For this review, take the finished solid that the model builds, in its own axes (mm). A direction names the side the tool comes from. Coordinates: 2 decimals unless noted, no trailing zeros. Write each loop counter-clockwise with the first axis right and the second up, starting at its lowest first coordinate (ties: lowest second). Pieces come first, ordered by that corner, then holes.
1) We need section C-C on z = 19. Give the number of separate pieces and of enclosed holes in the cut face, then the cut area to 3 significant figures.
2) We need section A-A on x = 13.5. Write out the cut boundary in (y, z).
3) Mouldability with a two-part tool opening along X and no side actions: class faces 4 (the face through (-28, 30.241, 12)), 5 (the face through (-17, 0, 69)), 6 (the face through (10.102, -12.325, 89.716)) as pulls with the +X half, pulls with the -X half, needs draft (parallel to the pull), parting line crosses it, or undercut.
4) Insertion check: P1, Ø8, axis at y = -30.5, z = 80.5, coming from the +X side; P2, Ø5.5, axis at y = 27.5, z = 18.5, coming from the +X side; P3, Ø3, axis at y = 24, z = 7, coming from the +X side; P4, Ø0.9, axis at x = -30.5, z = 13.5, coming from the +Y side. Each pin has a flat end and moves straight along its axis. Give the tip position at first contact, or say it passes through.
5) For faces 1 (the face through (-16.186, 25, 12)), 2 (the face through (8.91, -12.32, 36.75)), 3 (the face through (45.226, -17.865, 21.044)), list the 3-axis set-ups (+Z, -Z, +X, -X, +Y, -Y) from which the entire face can be reached by the end or side of a thin tool; tool diameter is ignored.
6) We need section D-D on x = -56.5. Write out the cut boundary in (y, z).
7) To check wall thickness, follow line 1 along Y through (x, z) = (-20.5, 15.5); line 2 along Y through (x, z) = (-66, 95); line 3 along Z through (x, y) = (0.5, 16). State the ranges of each line that lie inside material, in increasing order.
8) We need section B-B on y = -23. Write out the cut boundary in (x, z), then the cut area to 3 significant figures.
from build123d import *

# Parameters (mm, degrees)
F0_W     = 1.1385447797
F0_H     = 10.6680987737
F1_DEPTH = 25
F3_DEPTH = 25


with BuildPart() as f1:
    # F0 (on Top) → F1 (new body)
    with BuildSketch(Plane.XY):
        Polygon((0, -46.6304384172), (46.141307801, -17.2826088965), (-5.3850366841, -15.2486749252), align=None)
        Polygon((-32.335957761, 9.7168054916), (-37.6630462706, 40.7608710229), (-71.6585168016, 12.759203091), align=None)
        Polygon((46.141307801, -17.2826088965), (37.9891358316, 38.1521731615), (-9.3640666491, 7.9394637296), (-5.3850366841, -15.2486749252), align=None)
        Polygon((-5.3850366841, -15.2486749252), (-28.2065235078, -14.347827062), (-61.4673942327, -46.6304384172), (0, -46.6304384172), align=None)
        Polygon((-28.2065235078, -14.347827062), (-32.335957761, 9.7168054916), (-71.6585168016, 12.759203091), (-61.4673942327, -46.6304384172), align=None)
        Polygon((37.9891358316, 38.1521731615), (-37.6630462706, 40.7608710229), (-32.335957761, 9.7168054916), (-9.3640666491, 7.9394637296), align=None)
        Polygon((-29.9031199126, 24.5017413181), (-29.9031199126, 20.217390731), (-31.0679894271, 20.217390731), (-31.0679894271, 30.2405335024), (-25.4805644678, 30.2405335024), (-25.4805644678, 29.2050939339), (-29.9031199126, 29.2050939339), (-29.9031199126, 25.5371808865), (-25.7481992715, 25.5371808865), (-25.7481992715, 24.5017413181), align=None, mode=Mode.SUBTRACT)
        with BuildLine():
            Line((-18.5286407553, 20.217390731), (-19.3732259965, 20.217390731))
            Line((-19.3732259965, 20.217390731), (-19.5991799701, 21.2879299458))
            Line((-19.5991799701, 21.2879299458), (-19.6540231676, 21.2879299458))
            add(Edge.make_bspline(
                [(-19.6540231676, 21.2879299458), (-20.2156175098, 20.5815495622), (-20.7739212601, 20.3303677178)],
                knots=[0, 0, 0, 1, 1, 1], degree=2))
            add(Edge.make_bspline(
                [(-20.7739212601, 20.3303677178), (-21.3322250105, 20.0791858733), (-22.1702290679, 20.0791858733)],
                knots=[0, 0, 0, 1, 1, 1], degree=2))
            add(Edge.make_bspline(
                [(-22.1702290679, 20.0791858733), (-23.2868365686, 20.0791858733), (-23.9208239315, 20.6561363108)],
                knots=[0, 0, 0, 1, 1, 1], degree=2))
            add(Edge.make_bspline(
                [(-23.9208239315, 20.6561363108), (-24.5548112944, 21.2330867483), (-24.5548112944, 22.2948510515)],
                knots=[0, 0, 0, 1, 1, 1], degree=2))
            add(Edge.make_bspline(
                [(-24.5548112944, 22.2948510515), (-24.5548112944, 24.569746883), (-20.9154167096, 24.6794332779)],
                knots=[0, 0, 0, 1, 1, 1], degree=2))
            Line((-20.9154167096, 24.6794332779), (-19.6408608002, 24.721114108))
            Line((-19.6408608002, 24.721114108), (-19.6408608002, 25.1883781505))
            add(Edge.make_bspline(
                [(-19.6408608002, 25.1883781505), (-19.6408608002, 26.0724504939), (-20.0203757267, 26.4936462506)],
                knots=[0, 0, 0, 1, 1, 1], degree=2))
            add(Edge.make_bspline(
                [(-20.0203757267, 26.4936462506), (-20.3998906533, 26.9148420072), (-21.2378947108, 26.9148420072)],
                knots=[0, 0, 0, 1, 1, 1], degree=2))
            add(Edge.make_bspline(
                [(-21.2378947108, 26.9148420072), (-22.1768102516, 26.9148420072), (-23.3614233172, 26.3400852976)],
                knots=[0, 0, 0, 1, 1, 1], degree=2))
            Line((-23.3614233172, 26.3400852976), (-23.7124197811, 27.2109952736))
            add(Edge.make_bspline(
                [(-23.7124197811, 27.2109952736), (-23.1574066226, 27.5115359958), (-22.495997661, 27.6826467719)],
                knots=[0, 0, 0, 1, 1, 1], degree=2))
            add(Edge.make_bspline(
                [(-22.495997661, 27.6826467719), (-21.8345886994, 27.853757548), (-21.167695418, 27.853757548)],
                knots=[0, 0, 0, 1, 1, 1], degree=2))
            add(Edge.make_bspline(
                [(-21.167695418, 27.853757548), (-19.8251339437, 27.853757548), (-19.1768873495, 27.2581604234)],
                knots=[0, 0, 0, 1, 1, 1], degree=2))
            add(Edge.make_bspline(
                [(-19.1768873495, 27.2581604234), (-18.5286407553, 26.6625632988), (-18.5286407553, 25.3463265593)],
                knots=[0, 0, 0, 1, 1, 1], degree=2))
            Line((-18.5286407553, 25.3463265593), (-18.5286407553, 20.217390731))
        make_face(mode=Mode.SUBTRACT)
        with BuildLine():
            add(Edge.make_bspline(
                [(-15.0471945793, 26.7305688637), (-14.2530650798, 27.853757548), (-12.6889370877, 27.853757548)],
                knots=[0, 0, 0, 1, 1, 1], degree=2))
            add(Edge.make_bspline(
                [(-12.6889370877, 27.853757548), (-11.2081707557, 27.853757548), (-10.3888133854, 26.8424489865)],
                knots=[0, 0, 0, 1, 1, 1], degree=2))
            add(Edge.make_bspline(
                [(-10.3888133854, 26.8424489865), (-9.569456015, 25.831140425), (-9.569456015, 23.981827806)],
                knots=[0, 0, 0, 1, 1, 1], degree=2))
            add(Edge.make_bspline(
                [(-9.569456015, 23.981827806), (-9.569456015, 22.1303214591), (-10.3953945691, 21.1047536662)],
                knots=[0, 0, 0, 1, 1, 1], degree=2))
            add(Edge.make_bspline(
                [(-10.3953945691, 21.1047536662), (-11.2213331231, 20.0791858733), (-12.6889370877, 20.0791858733)],
                knots=[0, 0, 0, 1, 1, 1], degree=2))
            add(Edge.make_bspline(
                [(-12.6889370877, 20.0791858733), (-13.4238359339, 20.0791858733), (-14.030401698, 20.3501112689)],
                knots=[0, 0, 0, 1, 1, 1], degree=2))
            add(Edge.make_bspline(
                [(-14.030401698, 20.3501112689), (-14.6369674621, 20.6210366644), (-15.0471945793, 21.1848247345)],
                knots=[0, 0, 0, 1, 1, 1], degree=2))
            Line((-15.0471945793, 21.1848247345), (-15.1305562395, 21.1848247345))
            Line((-15.1305562395, 21.1848247345), (-15.3696725805, 20.217390731))
            Line((-15.3696725805, 20.217390731), (-16.185739359, 20.217390731))
            Line((-16.185739359, 20.217390731), (-16.185739359, 30.8854895047))
            Line((-16.185739359, 30.8854895047), (-15.0471945793, 30.8854895047))
            Line((-15.0471945793, 30.8854895047), (-15.0471945793, 28.2925031279))
            add(Edge.make_bspline(
                [(-15.0471945793, 28.2925031279), (-15.0471945793, 27.4215931519), (-15.1020377768, 26.7305688637)],
                knots=[0, 0, 0, 1, 1, 1], degree=2))
            Line((-15.1020377768, 26.7305688637), (-15.0471945793, 26.7305688637))
        make_face(mode=Mode.SUBTRACT)
        with BuildLine():
            Line((1.4342831273, 20.217390731), (0.5896978861, 20.217390731))
            Line((0.5896978861, 20.217390731), (0.3637439125, 21.2879299458))
            Line((0.3637439125, 21.2879299458), (0.308900715, 21.2879299458))
            add(Edge.make_bspline(
                [(0.308900715, 21.2879299458), (-0.2526936272, 20.5815495622), (-0.8109973775, 20.3303677178)],
                knots=[0, 0, 0, 1, 1, 1], degree=2))
            add(Edge.make_bspline(
                [(-0.8109973775, 20.3303677178), (-1.3693011279, 20.0791858733), (-2.2073051853, 20.0791858733)],
                knots=[0, 0, 0, 1, 1, 1], degree=2))
            add(Edge.make_bspline(
                [(-2.2073051853, 20.0791858733), (-3.323912686, 20.0791858733), (-3.9579000489, 20.6561363108)],
                knots=[0, 0, 0, 1, 1, 1], degree=2))
            add(Edge.make_bspline(
                [(-3.9579000489, 20.6561363108), (-4.5918874118, 21.2330867483), (-4.5918874118, 22.2948510515)],
                knots=[0, 0, 0, 1, 1, 1], degree=2))
            add(Edge.make_bspline(
                [(-4.5918874118, 22.2948510515), (-4.5918874118, 24.569746883), (-0.952492827, 24.6794332779)],
                knots=[0, 0, 0, 1, 1, 1], degree=2))
            Line((-0.952492827, 24.6794332779), (0.3220630824, 24.721114108))
            Line((0.3220630824, 24.721114108), (0.3220630824, 25.1883781505))
            add(Edge.make_bspline(
                [(0.3220630824, 25.1883781505), (0.3220630824, 26.0724504939), (-0.0574518441, 26.4936462506)],
                knots=[0, 0, 0, 1, 1, 1], degree=2))
            add(Edge.make_bspline(
                [(-0.0574518441, 26.4936462506), (-0.4369667707, 26.9148420072), (-1.2749708282, 26.9148420072)],
                knots=[0, 0, 0, 1, 1, 1], degree=2))
            add(Edge.make_bspline(
                [(-1.2749708282, 26.9148420072), (-2.213886369, 26.9148420072), (-3.3984994346, 26.3400852976)],
                knots=[0, 0, 0, 1, 1, 1], degree=2))
            Line((-3.3984994346, 26.3400852976), (-3.7494958985, 27.2109952736))
            add(Edge.make_bspline(
                [(-3.7494958985, 27.2109952736), (-3.19448274, 27.5115359958), (-2.5330737784, 27.6826467719)],
                knots=[0, 0, 0, 1, 1, 1], degree=2))
            add(Edge.make_bspline(
                [(-2.5330737784, 27.6826467719), (-1.8716648168, 27.853757548), (-1.2047715354, 27.853757548)],
                knots=[0, 0, 0, 1, 1, 1], degree=2))
            add(Edge.make_bspline(
                [(-1.2047715354, 27.853757548), (0.1377899389, 27.853757548), (0.7860365331, 27.2581604234)],
                knots=[0, 0, 0, 1, 1, 1], degree=2))
            add(Edge.make_bspline(
                [(0.7860365331, 27.2581604234), (1.4342831273, 26.6625632988), (1.4342831273, 25.3463265593)],
                knots=[0, 0, 0, 1, 1, 1], degree=2))
            Line((1.4342831273, 25.3463265593), (1.4342831273, 20.217390731))
        make_face(mode=Mode.SUBTRACT)
        with Locations((-7.0126661485, 25.5514401179)):
            Rectangle(F0_W, F0_H, mode=Mode.SUBTRACT)
        with BuildLine():
            add(Edge.make_bspline(
                [(4.9157293033, 26.7305688637), (5.7098588028, 27.853757548), (7.2739867949, 27.853757548)],
                knots=[0, 0, 0, 1, 1, 1], degree=2))
            add(Edge.make_bspline(
                [(7.2739867949, 27.853757548), (8.7547531269, 27.853757548), (9.5741104972, 26.8424489865)],
                knots=[0, 0, 0, 1, 1, 1], degree=2))
            add(Edge.make_bspline(
                [(9.5741104972, 26.8424489865), (10.3934678676, 25.831140425), (10.3934678676, 23.981827806)],
                knots=[0, 0, 0, 1, 1, 1], degree=2))
            add(Edge.make_bspline(
                [(10.3934678676, 23.981827806), (10.3934678676, 22.1303214591), (9.5675293135, 21.1047536662)],
                knots=[0, 0, 0, 1, 1, 1], degree=2))
            add(Edge.make_bspline(
                [(9.5675293135, 21.1047536662), (8.7415907595, 20.0791858733), (7.2739867949, 20.0791858733)],
                knots=[0, 0, 0, 1, 1, 1], degree=2))
            add(Edge.make_bspline(
                [(7.2739867949, 20.0791858733), (6.5390879487, 20.0791858733), (5.9325221846, 20.3501112689)],
                knots=[0, 0, 0, 1, 1, 1], degree=2))
            add(Edge.make_bspline(
                [(5.9325221846, 20.3501112689), (5.3259564205, 20.6210366644), (4.9157293033, 21.1848247345)],
                knots=[0, 0, 0, 1, 1, 1], degree=2))
            Line((4.9157293033, 21.1848247345), (4.8323676432, 21.1848247345))
            Line((4.8323676432, 21.1848247345), (4.5932513021, 20.217390731))
            Line((4.5932513021, 20.217390731), (3.7771845236, 20.217390731))
            Line((3.7771845236, 20.217390731), (3.7771845236, 30.8854895047))
            Line((3.7771845236, 30.8854895047), (4.9157293033, 30.8854895047))
            Line((4.9157293033, 30.8854895047), (4.9157293033, 28.2925031279))
            add(Edge.make_bspline(
                [(4.9157293033, 28.2925031279), (4.9157293033, 27.4215931519), (4.8608861058, 26.7305688637)],
                knots=[0, 0, 0, 1, 1, 1], degree=2))
            Line((4.8608861058, 26.7305688637), (4.9157293033, 26.7305688637))
        make_face(mode=Mode.SUBTRACT)
        Polygon((-9.3640666491, 7.9394637296), (-32.335957761, 9.7168054916), (-28.2065235078, -14.347827062), (-5.3850366841, -15.2486749252), align=None)
    extrude(amount=F1_DEPTH)

    # F2 (on Front) → F3 (join)
    with BuildSketch(Plane.XZ):
        Polygon((-17.7594870329, 106.7427992821), (-75.7184699178, 110.903725028), (-59.3579299748, 76.7451450229), (-34.2380218208, 51.2733086944), (-3.0318840951, 35.7375395996), (21.1975596517, 37.7931054263), (47.9272156954, 3.3937320113), (40.3265580535, 36.2278595567), (37.193346135, 73.1597743332), align=None)
    extrude(amount=F3_DEPTH)


solid = f1.part
Result:
1. separate pieces: 1
1. enclosed holes: 6
1. area: 8,340 mm2
2. outline: (-38.04, 0) - (39, 0) - (39, 25) - (-38.04, 25) - close; (-25, 37.14) - (0, 37.14) - (0, 87.64) - (-25, 87.64) - close
3. face 4: undercut
3. face 5: needs draft
3. face 6: pulls with the +X half
4. P1: passes through
4. P2: stops at x = 39.96
4. P3: stops at x = 40.29
4. P4: stops at y = 40.53
5. face 1: +Z, -Z
5. face 2: +Y, -Y
5. face 3: +Z, +X, -Y
6. outline: (-46.63, 0) - (25.25, 0) - (25.25, 25) - (-46.63, 25) - close; (-25, 73.85) - (0, 73.85) - (0, 109.52) - (-25, 109.52) - close
7. line 1: y = -46.63 to 20.48, 24.69 to 26.8, 27.81 to 40.17
7. line 2: y = -25 to 0
7. line 3: z = 0 to 25
8. outline: (-75.72, 110.9) - (-59.36, 76.75) - (-34.24, 51.27) - (-3.03, 35.74) - (21.2, 37.79) - (31.14, 25) - (-65.52, 25) - (-65.52, 0) - (37.15, 0) - (37.15, 17.26) - (47.93, 3.39) - (40.33, 36.23) - (37.19, 73.16) - (-17.76, 106.74) - close
8. area: 8,170 mm2
